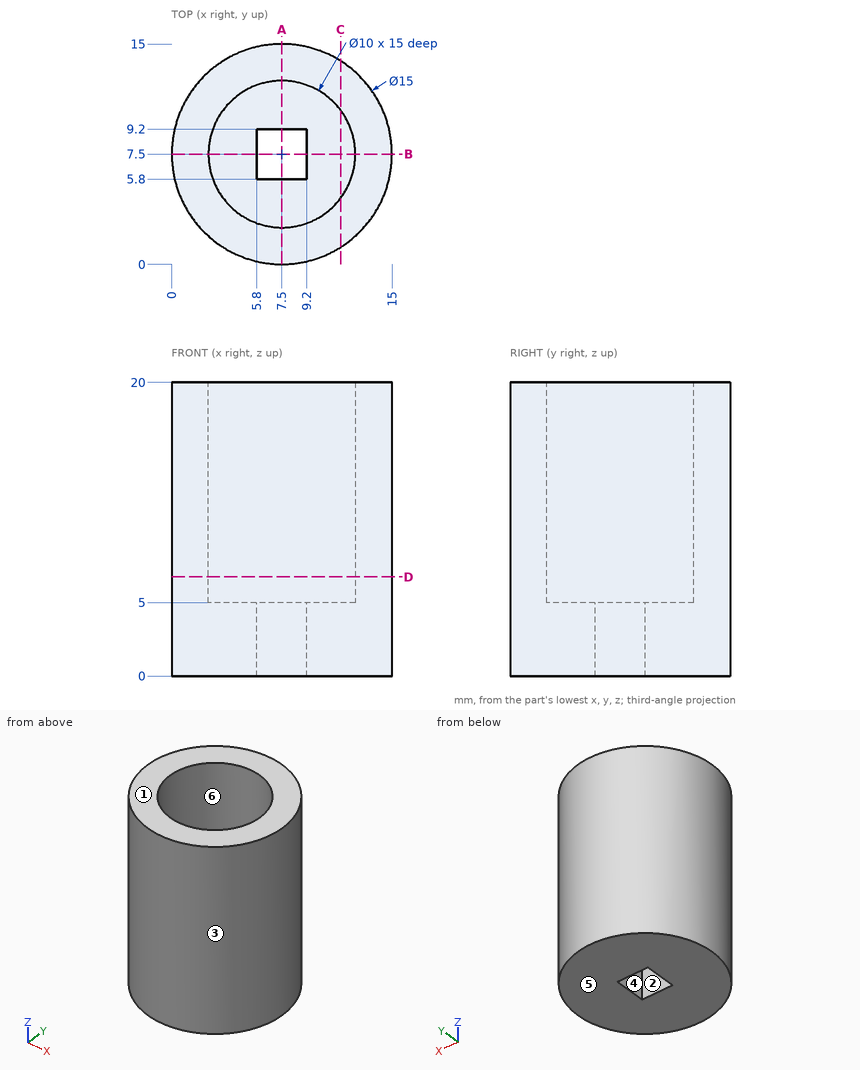
Input: dimensioned drawing with shaded views. Units: mm. Origin: part minimum x, y, z. A direction names the side the tool comes from. Give positions to 0.01 mm unless a question says otherwise; leave off trailing zeros. Write each loop counter-clockwise with the first axis right and the second up, starting at its lowest first coordinate (ties: lowest second). Pieces come first, ordered by that corner, then holes. Notation, with made-up numbers: (87.25, 30.5) -> (124.25, 30.5) arc R30 cw to (124.25, 63.5) -> close; hole circle Ø9 at (23, -20.5). An arc over 180 degrees is marked (long way). Return JSON: item names as keys, results as strings. Group by question number.
1. Section C-C, the plane x = 11.5. Output: boundary loops of the cut face in (y, z), then the cut area to 3 significant figures.
2. Access query for the marked faces 1 and 2. Directions: +Z, -Z, +X, -X, +Y, -Y. A direction counts if a zero-diameter tool reaches every point of the face in a straight line with its end or side. Return the directions, or none.
3. Section D-D, the plane z = 6.75. Output: boundary loops of the cut face in (x, y), then the cut area to 3 significant figures.
4. Mould query, pull axis X, two halves, no side actions, for the marked faces 3, 4, 5 and 6. Classes: +X half, -X half, draft (parallel to the pull), parting line (faces both ways), or undercut.
5. Section A-A, the plane x = 7.5. Output: boundary loops of the cut face in (y, z).
6. Pin query (flat end, axial travel): pin 1 Ø1 at (y, z) = (2, 3.5) entering from -X; pin 2 Ø1 at (y, z) = (3.5, 9.5) entering from -X; pin 3 Ø1.5 at (x, z) = (5, 3.5) entering from -Y. Return the tip coordinate at first contact, or that it passes through.
7. Material intervals for line 1 (Y direction, x = 7.5, z = 12.25); line 2 (Z direction, x = 4, y = 5); line 3 (X direction, y = 9.5, z = 13.5), sorted ascending. Write a range as from..to.
Determined:
{
 "1": {"outline": "(1.16, 0) -> (13.84, 0) -> (13.84, 20) -> (10.5, 20) -> (10.5, 5) -> (4.5, 5) -> (4.5, 20) -> (1.16, 20) -> close", "area": "164 mm2"},
 "2": {"face 1": "+Z, +X, -X, +Y, -Y", "face 2": "+Z, -Z"},
 "3": {"outline": "circle Ø15 at (7.5, 7.5); hole circle Ø10 at (7.5, 7.5)", "area": "98.2 mm2"},
 "4": {"face 3": "parting line", "face 4": "undercut", "face 5": "draft", "face 6": "undercut"},
 "5": {"outline": "(0, 0) -> (5.8, 0) -> (5.8, 5) -> (2.5, 5) -> (2.5, 20) -> (0, 20) -> close; (9.2, 0) -> (15, 0) -> (15, 20) -> (12.5, 20) -> (12.5, 5) -> (9.2, 5) -> close"},
 "6": {"pin 1": "stops at x = 1.91", "pin 2": "stops at x = 0.87", "pin 3": "stops at y = 0.21"},
 "7": {"line 1": "y = 0..2.5, 12.5..15", "line 2": "z = 0..5", "line 3": "x = 0.27..2.92, 12.08..14.73"}
}
